Verification items for the finished model (mm, model axes). Face numbers are marked on the shaded views. A direction names the side the tool comes from. Coordinates: 2 decimals unless noted, no trailing zeros. Write each loop counter-clockwise with the first axis right and the second up, starting at its lowest first coordinate (ties: lowest second). Pieces come first, ordered by that corner, then holes. Notation, with made-up numbers: (76.25, -19) -> (130.25, -19) arc R33 cw to (130.25, 15) -> close; hole circle Ø9 at (13, 18.5). An arc over 180 degrees is marked (long way). Answer in a Markdown table with one row per item.
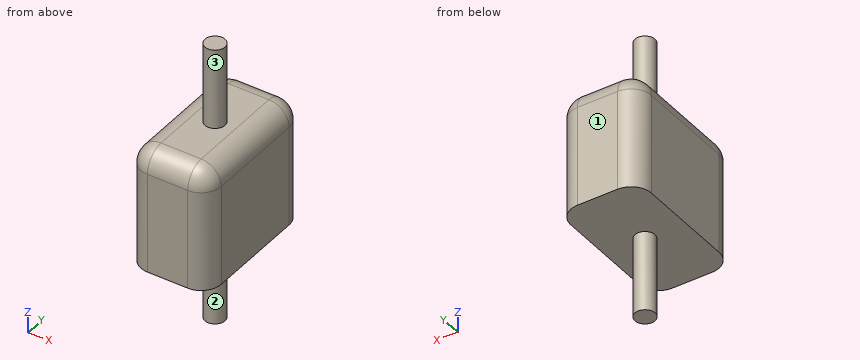
```python
from build123d import *

# Parameters (mm, degrees)
F0_W     = 20
F0_H     = 35
F1_DEPTH = 30
F2_R     = 2.5
F3_DEPTH = 20
F4_R     = 5
F5_R     = 2.5
F6_DEPTH = 20


with BuildPart() as f1:
    # F0 (on Top) → F1 (new body)
    with BuildSketch(Plane.XY):
        Rectangle(F0_W, F0_H)
    extrude(amount=F1_DEPTH)

    # F2 (on face) → F3 (join)
    with BuildSketch(Plane.XY.offset(30)):
        Circle(F2_R)
    extrude(amount=F3_DEPTH)

    # F4
    f4_edges = [f1.edges().sort_by_distance(p)[0] for p in [
        (0, -17.5, 30),
        (10, -17.5, 15),
        (-10, -17.5, 15),
        (-10, 0, 30),
        (0, 17.5, 30),
        (10, 0, 30),
        (10, 17.5, 15),
        (-10, 17.5, 15),
    ]]
    fillet(f4_edges, radius=F4_R)

    # F5 (on face) → F6 (join)
    with BuildSketch(Plane(origin=(0, 0, 0), x_dir=(1, 0, 0), z_dir=(0, 0, -1))):
        Circle(F5_R)
    extrude(amount=F6_DEPTH)


solid = f1.part
```
1. Depth check by flat-ended pin: P1, Ø1, axis at x = 5, y = 13.5, coming from the +Z side; P2, Ø6, axis at x = -7.5, z = 31, coming from the -Y side. Enter the tip coordinate at first touch or a pass-through.
Geometry says:
| item | result |
|---|---|
| P1 | z = 29.97 |
| P2 | y = -16.07 |
2. Section check B-B, the plane z = 22.5. Record the boundary of the cut face in (x, y), plus the area to 3 significant figures.
Geometry says:
| item | result |
|---|---|
| outline | (-10, -12.5) arc R5 ccw to (-5, -17.5) -> (5, -17.5) arc R5 ccw to (10, -12.5) -> (10, 12.5) arc R5 ccw to (5, 17.5) -> (-5, 17.5) arc R5 ccw to (-10, 12.5) -> close |
| area | 679 mm^2 |
3. Thickness scan on line 1 (Z direction, x = -3.5, y = 2); line 2 (Y direction, x = 5.75, z = 24); line 3 (Z direction, x = -8, y = 1.5). Record the ranges inside material, lowest first. Write a range as from..to.
Geometry says:
| item | result |
|---|---|
| line 1 | 0..30 |
| line 2 | -17.44..17.44 |
| line 3 | 0..29 |
4. Section check C-C, the plane x = 0. Record the boundary of the cut face in (y, z), plus the area to 3 significant figures.
Geometry says:
| item | result |
|---|---|
| outline | (-17.5, 0) -> (-2.5, 0) -> (-2.5, -20) -> (2.5, -20) -> (2.5, 0) -> (17.5, 0) -> (17.5, 25) arc R5 ccw to (12.5, 30) -> (2.5, 30) -> (2.5, 50) -> (-2.5, 50) -> (-2.5, 30) -> (-12.5, 30) arc R5 ccw to (-17.5, 25) -> close |
| area | 1,240 mm^2 |
5. Tool access check on the marked faces 1, 2 and 3. Record the directions out of +Z, -Z, +X, -X, +Y, -Y that give a thin tool (end or side, any length) a straight path to the whole face; none if there is none.
Geometry says:
| item | result |
|---|---|
| face 1 | +Z, -Z, +X, -X, +Y |
| face 2 | -Z |
| face 3 | +Z |
6. Section check D-D, the plane y = 0. Record the boundary of the cut face in (x, z), plus the area to 3 significant figures.
Geometry says:
| item | result |
|---|---|
| outline | (-10, 0) -> (-2.5, 0) -> (-2.5, -20) -> (2.5, -20) -> (2.5, 0) -> (10, 0) -> (10, 25) arc R5 ccw to (5, 30) -> (2.5, 30) -> (2.5, 50) -> (-2.5, 50) -> (-2.5, 30) -> (-5, 30) arc R5 ccw to (-10, 25) -> close |
| area | 789 mm^2 |
7. Section check A-A, the plane y = 6. Record the boundary of the cut face in (x, z).
Geometry says:
| item | result |
|---|---|
| outline | (-10, 0) -> (10, 0) -> (10, 25) arc R5 ccw to (5, 30) -> (-5, 30) arc R5 ccw to (-10, 25) -> close |
